The model under review builds one solid part; all positions refer to its coordinate system, in mm. Face numbers are marked on the shaded views. Coordinates: 2 decimals unless noted, no trailing zeros. Order: outer loops, then holes, each group sorted by start corner. A loop starts at its lowest first (then second) coordinate and runs counter-clockwise, first axis right, second up. Notation, with made-up numbers: (-39, 34.5) -> (-34, 34.5) arc R6 ccw to (-34, 45.5) -> close; hole circle Ø6 at (3, -31.75). An arc over 180 degrees is marked (long way). Use one line per item in the form item = value. Start each with the question number.
(1) Take a section at C-C (z = -16.5). State the section outline as (x, y) points.
(2) Insertion check: pin 1 Ø2.5 at (x, z) = (37.5, -13.5) entering from +Y; pin 2 Ø3 at (x, z) = (5, -18.5) entering from -Y. Each pin has a flat end and moves straight along its axis. Give the tip position at first contact, or say it passes through.
(3) Take a section at B-B (y = 1.35). State the section outline as (x, z) points.
(4) Mouldability with a two-part tool opening along Z and no side actions: class the marked faces 1 and 2 as +Z half, -Z half, draft (parallel to the pull), parting line (faces both ways), or undercut.
(5) Take a section at A-A (z = -13). State the section outline as (x, y) points, then the cut area to 3 significant figures.
(6) Wall thickness on line 1 along X through (y, z) = (0.85, -13); line 2 along Z through (x, y) = (40, 1.4); line 3 along Y through (x, z) = (42, -15): over which ranges is each line inside the solid? List them lowest first.
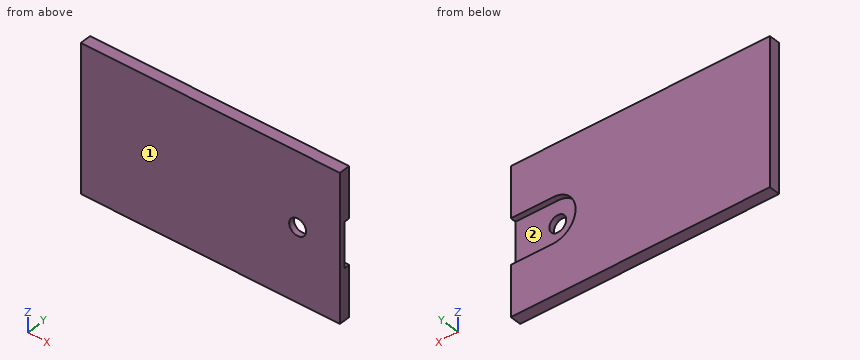
```python
from build123d import *

# Parameters (mm, degrees)
SKETCH1_W                           = 46
SKETCH1_H                           = 26
BOSS_EXTRUDE1_DEPTH                 = 2
CUT_EXTRUDE1_DEPTH                  = 1
F_3_0MM_DOWEL_HOLE1_D               = 3
F_3_0MM_DOWEL_HOLE1_DEPTH           = 1
F_3_0MM_DOWEL_HOLE1_ON_FACE_2_D     = 3
F_3_0MM_DOWEL_HOLE1_ON_FACE_2_DEPTH = 1


with BuildPart() as part:
    # Sketch1 → Boss-Extrude1 (new body)
    with BuildSketch(Plane(origin=(0, 0, 0), x_dir=(1, 0, 0), z_dir=(0, 1, 0))):
        with Locations((23, 13)):
            Rectangle(SKETCH1_W, SKETCH1_H)
    extrude(amount=BOSS_EXTRUDE1_DEPTH)

    # Sketch2 → Cut-Extrude1 (cut)
    with BuildSketch(Plane(origin=(0, 2, 0), x_dir=(1, 0, 0), z_dir=(0, 1, 0))):
        with BuildLine():
            Line((38.5, 17), (53.5, 17))
            ThreePointArc((53.5, 17), (57.5, 13), (53.5, 9))
            Line((53.5, 9), (38.5, 9))
            ThreePointArc((38.5, 9), (34.5, 13), (38.5, 17))
        make_face()
    extrude(amount=-CUT_EXTRUDE1_DEPTH, mode=Mode.SUBTRACT)

    # Ø3.0mm Dowel Hole1
    with Locations(Plane(origin=(38.5, 1, -13), x_dir=(0, 0, 1), z_dir=(0, 1, 0))):
        with Locations((0, 0)):
            Hole(F_3_0MM_DOWEL_HOLE1_D / 2, depth=F_3_0MM_DOWEL_HOLE1_DEPTH)

    # Ø3.0mm Dowel Hole1 on face 2
    with Locations(Plane(origin=(65.15789834, 32.144542586, 0), x_dir=(0, 0, 1), z_dir=(0, 1, 0))):
        with Locations((0, 0)):
            Hole(F_3_0MM_DOWEL_HOLE1_ON_FACE_2_D / 2, depth=F_3_0MM_DOWEL_HOLE1_ON_FACE_2_DEPTH)


solid = part.part
```
Findings:
q1.outline = (0, 0) -> (46, 0) -> (46, 1) -> (36.56, 1) -> (36.56, 2) -> (0, 2) -> close
q2.pin_1 = 1
q2.pin_2 = 0
q3.outline = (0, -26) -> (46, -26) -> (46, -17) -> (38.5, -17) arc R4 cw to (38.5, -9) -> (46, -9) -> (46, 0) -> (0, 0) -> close
q4.face_1 = draft
q4.face_2 = undercut
q5.outline = (0, 0) -> (37, 0) -> (37, 1) -> (34.5, 1) -> (34.5, 2) -> (0, 2) -> close; (40, 0) -> (46, 0) -> (46, 1) -> (40, 1) -> close
q5.area = 77.5 mm²
q6.line_1 = 0 to 37, 40 to 46
q6.line_2 = -26 to -17, -9 to 0
q6.line_3 = 0 to 1
